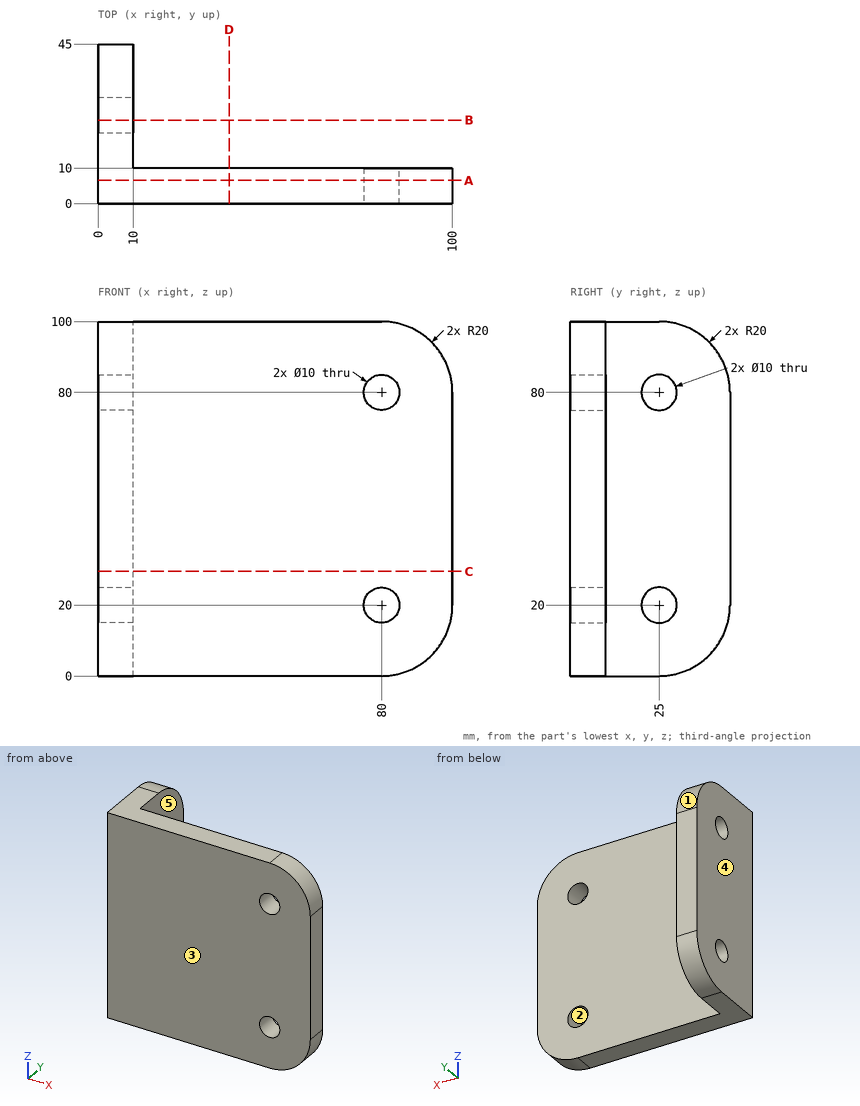
Design review of the part shown in the three views and the two pictorial views. Dimensions are in mm from the part's minimum x, y and z. A direction names the side the tool comes from. Round coordinates to 2 decimals unless told otherwise and drop trailing zeros. Write each loop counter-clockwise with the first axis right and the second up, starting at its lowest first coordinate (ties: lowest second). Pieces come first, ordered by that corner, then holes. Notation, with made-up numbers: M 15.5,9 L 71.5,9 A26 ccw 71.5,41 Z; hole C -25.75,72.5 d9. An arc over 180 degrees is marked long. One line per item, written item: value. Start each with the question number.
1. Take a section at D-D on x = 37. State the section outline as (y, z) points.
2. Clearance check with flat-ended pins moving along their axes: P1, Ø16, axis at y = 25, z = 80, coming from the -X side; P2, Ø9, axis at y = 25, z = 20, coming from the +X side; P3, Ø13, axis at x = 80, z = 80, coming from the +Y side; P4, Ø10.5, axis at y = 21.5, z = 62, coming from the +X side. State where each tip first meets the part, or that it passes through.
3. For the marked faces 4 and 5, list the 3-axis set-ups (+Z, -Z, +X, -X, +Y, -Y) from which the entire face can be reached by the end or side of a thin tool; tool diameter is ignored.
4. Take a section at B-B on y = 23.5. State the section outline as (x, z) points.
5. Take a section at A-A on y = 6.5. State the section outline as (x, z) points.
6. Take a section at C-C on z = 29.5. State the section outline as (x, y) points.
7. To check wall thickness, follow probe 1 along Z at (x, y) = (80, 8); probe 2 along Y at (x, z) = (6, 20); probe 3 along Y at (x, z) = (58, 19). State the ranges of each line that lie inside material, in increasing order. Write a range as from..to.
8. Draft analysis for pull direction Z (two halves, no side actions). For the marked faces 1, 2 and 3, state which applies: pulls with the +Z half, pulls with the -Z half, needs draft (parallel to the pull), parting line crosses it, or undercut.
Computed:
1. outline: M 0,0 L 10,0 L 10,100 L 0,100 Z
2. P1: stops at x = 0
2. P2: passes through
2. P3: stops at y = 10
2. P4: stops at x = 10
3. face 4: +Z, -Z, -X, +Y, -Y
3. face 5: +Z, -Z, +X, +Y
4. outline: M 0,0 L 10,0 L 10,15.23 L 0,15.23 Z; M 0,24.77 L 10,24.77 L 10,75.23 L 0,75.23 Z; M 0,84.77 L 10,84.77 L 10,100 L 0,100 Z
5. outline: M 0,0 L 80,0 A20 ccw 100,20 L 100,80 A20 ccw 80,100 L 0,100 Z; hole C 80,20 d10; hole C 80,80 d10
6. outline: M 0,0 L 100,0 L 100,10 L 10,10 L 10,45 L 0,45 Z
7. probe 1: z = 0..15, 25..75, 85..100
7. probe 2: y = 0..20, 30..45
7. probe 3: y = 0..10
8. face 1: pulls with the +Z half
8. face 2: undercut
8. face 3: needs draft
